The model under review builds one solid part; all positions refer to its coordinate system, in mm. Face numbers are marked on the shaded views. A direction names the side the tool comes from. Coordinates: 2 decimals unless noted, no trailing zeros. Write each loop counter-clockwise with the first axis right and the second up, starting at its lowest first coordinate (ties: lowest second). Pieces come first, ordered by that corner, then holes. Notation, with made-up numbers: (-18, -13.5) - (26, -13.5) arc R26 cw to (26, 5.5) - close; hole circle Ø7 at (-7.5, 19). An arc over 180 degrees is marked (long way). Return JSON: item names as keys, results as strings. Group by question number.
(1) For pin 1 Ø0.6 at (x, y) = (3, -1) entering from +Z; pin 2 Ø1.8 at (x, z) = (3, -4.5) entering from -Y; pin 3 Ø3 at (x, z) = (4, -3.75) entering from -Y, all flat-tipped, find the tip position at first contact; note any pin that passes through.
(2) Tool access review of the marked faces 1, 2 and 3: name each direction out of +Z, -Z, +X, -X, +Y, -Y from which nothing blocks a thin tool from reaching the whole face with its end or side.
(3) Draft analysis for pull direction X (two halves, no side actions). For the marked faces 4, 5 and 6, state which applies: released by +X, released by -X, zero draft, split by the parting line, or undercut.
(4) We need section B-B on y = 0.45. State the section outline as (x, z) points, then the cut area to 3 significant figures.
(5) We need section C-C on z = -4. State the section outline as (x, y) points.
(6) To check wall thickness, follow L1, parallel to Y at x = 2.25, z = -6; L2, parallel to Y at x = 5.5, z = -3.25; L3, parallel to X at y = 0.6, z = -3.75. State the ranges of each line that lie inside material, in increasing order. Write a range as from..to.
(7) We need section D-D on y = 2.4. State the section outline as (x, z) points.
(8) We need section A-A on x = 4. State the section outline as (y, z) points.
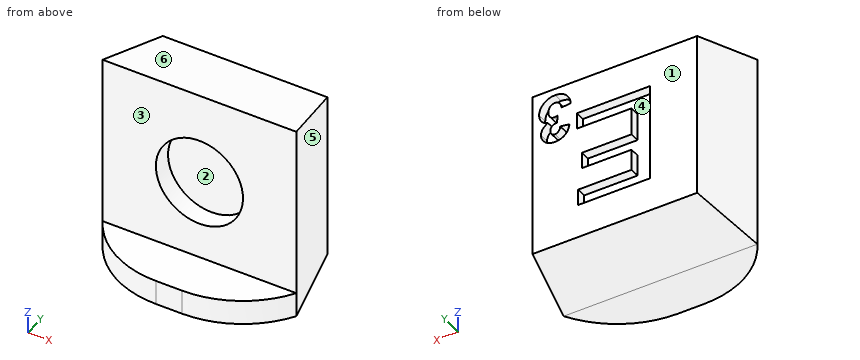
```python
from build123d import *

# Parameters (mm, degrees)
SKETCH1_W               = 8
SKETCH1_H               = 8
BOSS_EXTRUDE1_DEPTH     = 3
CUT_EXTRUDE1_DEPTH      = 12.704699911
CUT_EXTRUDE1_DEPTH_BACK = 12.704699911
CUT_EXTRUDE2_DEPTH      = 11
SKETCH4_R               = 1.8
CUT_EXTRUDE3_DEPTH      = 0.8
SKETCH5_W               = 8
SKETCH5_H               = 1
BOSS_EXTRUDE2_DEPTH     = 2
FILLET1_R               = 4
CUT_EXTRUDE4_DEPTH      = 0.4
CUT_EXTRUDE5_DEPTH      = 0.4


with BuildPart() as part:
    # Sketch1 → Boss-Extrude1 (new body)
    with BuildSketch(Plane(origin=(0, 0, 0), x_dir=(1, 0, 0), z_dir=(0, 1, 0))):
        with Locations((4, 4)):
            Rectangle(SKETCH1_W, SKETCH1_H)
    extrude(amount=BOSS_EXTRUDE1_DEPTH)

    # Sketch2 → Cut-Extrude1 (cut, two sides: drawn at the far end of the back side and taken through both)
    with BuildSketch(Plane.XY.offset(-CUT_EXTRUDE1_DEPTH_BACK)):
        Polygon((0, 0), (0.6, 3), (0, 3), align=None)
        Polygon((8, 0), (7.4, 3), (8, 3), align=None)
    extrude(amount=CUT_EXTRUDE1_DEPTH + CUT_EXTRUDE1_DEPTH_BACK, mode=Mode.SUBTRACT)

    # Sketch3 → Cut-Extrude2 (cut)
    with BuildSketch(Plane(origin=(0, 0, 0), x_dir=(0, 0, -1), z_dir=(1, 0, 0))):
        Polygon((0, 0), (0.6, 3), (0, 3), align=None)
        Polygon((8, 3), (7.4, 3), (8, 0), align=None)
    extrude(amount=CUT_EXTRUDE2_DEPTH, mode=Mode.SUBTRACT)

    # Sketch4 → Cut-Extrude3 (cut)
    with BuildSketch(Plane.XZ):
        with Locations(Location((4, -3.75, 0), (0, 0, 270))):
            Circle(SKETCH4_R)
    extrude(amount=-CUT_EXTRUDE3_DEPTH, mode=Mode.SUBTRACT)

    # Sketch5 → Boss-Extrude2 (add)
    with BuildSketch(Plane.XZ):
        with Locations((4, -7.5)):
            Rectangle(SKETCH5_W, SKETCH5_H)
    extrude(amount=BOSS_EXTRUDE2_DEPTH)

    # Fillet1
    # the kernel refuses this fillet: 4 mm, written as the material it takes off along each edge
    with BuildSketch(Plane(origin=(8, -2, -16.660254038), x_dir=(0, 1, 0), z_dir=(0, 0, 1)), Plane(origin=(0, -2, 1.660254038), x_dir=(0, 1, 0), z_dir=(0, 0, -1))) as fillet1_piece_1:
        with BuildLine():
            CenterArc((4, 3.464101615), FILLET1_R, 180, 60)
            Line((0, 3.464101615), (-0.08, 3.464101615))
            Line((-0.08, 3.464101615), (-0.08, 0))
            Line((-0.08, 0), (0, -0.08))
            ThreePointArc((0, -0.08), (1, -0.08), (1.96, -0.069282032))
            Line((1.96, -0.069282032), (2, 0))
        make_face()
    extrude(amount=18.320508076, mode=Mode.SUBTRACT)

    # Sketch6 → Cut-Extrude4 (cut)
    with BuildSketch(Plane(origin=(0, 3, 0), x_dir=(1, 0, 0), z_dir=(0, 1, 0))):
        Polygon((2.544225106, 2.010567225), (2.544225106, 6.010567225), (5.51858408, 6.010567225), (5.51858408, 5.343900558), (3.313455875, 5.343900558), (3.313455875, 4.472105686), (5.364737926, 4.472105686), (5.364737926, 3.80543902), (3.313455875, 3.80543902), (3.313455875, 2.677233891), (5.569866131, 2.677233891), (5.569866131, 2.010567225), align=None)
    extrude(amount=-CUT_EXTRUDE4_DEPTH, mode=Mode.SUBTRACT)

    # Sketch7 → Cut-Extrude5 (cut)
    with BuildSketch(Plane(origin=(0, 3, 0), x_dir=(1, 0, 0), z_dir=(0, 1, 0))):
        with BuildLine():
            Line((5.822088817, 1.468310464), (6.206704202, 1.515586105))
            add(Edge.make_bspline(
                [(6.206704202, 1.515586105), (6.210025755, 1.491936921), (6.21633053, 1.447047438), (6.235989072, 1.384914698), (6.261652315, 1.330845836), (6.295629161, 1.286544364), (6.334912115, 1.251310519), (6.37872169, 1.226169889), (6.426661607, 1.210315729), (6.460052531, 1.208713548), (6.477136894, 1.207893797)],
                knots=[0, 0, 0, 0, 1.26631894, 2.403651751, 3.447242243, 4.428907923, 5.348362865, 6.231623936, 7.095215805, 8, 8, 8, 8], degree=3))
            add(Edge.make_bspline(
                [(6.477136894, 1.207893797), (6.486366298, 1.208091994), (6.504648304, 1.20848459), (6.531523321, 1.212603697), (6.557345996, 1.219374529), (6.58186155, 1.229117251), (6.605187017, 1.241222715), (6.627629553, 1.255638676), (6.648246393, 1.273643613), (6.668375088, 1.29334292), (6.68623752, 1.315767324), (6.701972196, 1.340096861), (6.715784117, 1.366090219), (6.726489771, 1.394417604), (6.734869896, 1.424465406), (6.740860884, 1.456364057), (6.744506994, 1.489993317), (6.74494315, 1.513039367), (6.74516574, 1.524800849)],
                knots=[0, 0, 0, 0, 0.951760839, 1.885289532, 2.797832748, 3.70117291, 4.60103766, 5.506897018, 6.445598779, 7.420035506, 8.410036365, 9.396193293, 10.407074535, 11.440988179, 12.514285005, 13.622404236, 14.786601276, 16, 16, 16, 16], degree=3))
            add(Edge.make_bspline(
                [(6.74516574, 1.524800849), (6.744331981, 1.546629456), (6.742741494, 1.588269906), (6.730451294, 1.647346431), (6.709137892, 1.699277092), (6.679276772, 1.743130281), (6.643793264, 1.778406879), (6.604044422, 1.8049236), (6.559654571, 1.820157256), (6.528795478, 1.822230353), (6.513194586, 1.823278413)],
                knots=[0, 0, 0, 0, 1.241512862, 2.368321189, 3.414110003, 4.41529485, 5.36642979, 6.245396713, 7.112955941, 8, 8, 8, 8], degree=3))
            add(Edge.make_bspline(
                [(6.513194586, 1.823278413), (6.502087722, 1.822994208), (6.47854234, 1.822391724), (6.441918774, 1.81613185), (6.401980616, 1.80749294), (6.374785766, 1.799182881), (6.360550356, 1.7948329)],
                knots=[0, 0, 0, 0, 0.854525515, 1.811503923, 2.854410343, 4, 4, 4, 4], degree=3))
            Line((6.360550356, 1.7948329), (6.396608048, 2.105329695))
            add(Edge.make_bspline(
                [(6.396608048, 2.105329695), (6.407296254, 2.105146348), (6.428036665, 2.104790564), (6.458323888, 2.107301653), (6.486673662, 2.111886341), (6.513019839, 2.119324972), (6.53738695, 2.128349551), (6.559988104, 2.139688262), (6.580270378, 2.153798702), (6.604965361, 2.175098338), (6.630230561, 2.207014566), (6.6530719, 2.250778884), (6.665798637, 2.300679459), (6.667408863, 2.335629458), (6.668242663, 2.353727131)],
                knots=[0, 0, 0, 0, 0.916749589, 1.778948191, 2.604102396, 3.376994206, 4.124053722, 4.831292757, 5.54010828, 6.238660037, 7.62386988, 9.002523041, 10.447858069, 12, 12, 12, 12], degree=3))
            add(Edge.make_bspline(
                [(6.668242663, 2.353727131), (6.667680515, 2.36913782), (6.666602635, 2.398686702), (6.656933325, 2.440733393), (6.640429824, 2.477855418), (6.617345194, 2.50940841), (6.589028098, 2.535030406), (6.555929861, 2.553963194), (6.518019093, 2.565003531), (6.491366313, 2.566231188), (6.477537535, 2.566868156)],
                knots=[0, 0, 0, 0, 1.146968804, 2.199229744, 3.192297141, 4.153502289, 5.090509175, 6.0173182, 6.971286811, 8, 8, 8, 8], degree=3))
            add(Edge.make_bspline(
                [(6.477537535, 2.566868156), (6.463673911, 2.566182836), (6.436422829, 2.564835732), (6.397428508, 2.551510744), (6.361454157, 2.530893795), (6.329709376, 2.501368407), (6.302195486, 2.464646404), (6.280874208, 2.419861118), (6.265858745, 2.367714197), (6.260698213, 2.33018187), (6.257986253, 2.3104579)],
                knots=[0, 0, 0, 0, 0.889956214, 1.749345552, 2.62404616, 3.543272128, 4.520224035, 5.562553653, 6.719074424, 8, 8, 8, 8], degree=3))
            Line((6.257986253, 2.3104579), (5.873370869, 2.368150208))
            add(Edge.make_bspline(
                [(5.873370869, 2.368150208), (5.879712758, 2.397514751), (5.891852554, 2.453725064), (5.916656, 2.532479948), (5.945759151, 2.602002338), (5.979761878, 2.663071325), (6.020038823, 2.716762155), (6.067859884, 2.763365742), (6.122509575, 2.804234412), (6.183883545, 2.838478774), (6.250614825, 2.865925856), (6.321633047, 2.886240153), (6.396757082, 2.897882068), (6.448117417, 2.899417689), (6.474332407, 2.90020149)],
                knots=[0, 0, 0, 0, 1.220808349, 2.336900656, 3.3513467, 4.279992853, 5.171472476, 6.069835959, 6.985198729, 7.938095762, 8.919113729, 9.91246339, 10.934493858, 12, 12, 12, 12], degree=3))
            add(Edge.make_bspline(
                [(6.474332407, 2.90020149), (6.496795991, 2.899690329), (6.540685792, 2.898691614), (6.604687523, 2.890097866), (6.665244055, 2.876137228), (6.722439804, 2.856388937), (6.776539911, 2.831244798), (6.826641223, 2.799609265), (6.873794781, 2.763093379), (6.901724377, 2.73467508), (6.915838817, 2.720313669)],
                knots=[0, 0, 0, 0, 1.096978699, 2.143298912, 3.148181587, 4.128190255, 5.094201205, 6.055441919, 7.017302331, 8, 8, 8, 8], degree=3))
            add(Edge.make_bspline(
                [(6.915838817, 2.720313669), (6.926741328, 2.708075606), (6.948274918, 2.683904162), (6.976233385, 2.645150995), (6.999633117, 2.604882958), (7.019482141, 2.563940258), (7.034243104, 2.52137348), (7.04524752, 2.477850813), (7.051783755, 2.43298662), (7.05249893, 2.402626167), (7.052858048, 2.387380977)],
                knots=[0, 0, 0, 0, 1.065582675, 2.104636323, 3.101288825, 4.092056841, 5.059084899, 6.026073946, 7.008813224, 8, 8, 8, 8], degree=3))
            add(Edge.make_bspline(
                [(7.052858048, 2.387380977), (7.052074688, 2.365937591), (7.050530541, 2.323668734), (7.036361111, 2.262180096), (7.013586987, 2.204054017), (6.982096895, 2.149068456), (6.941041129, 2.097733658), (6.890499978, 2.050511525), (6.831958555, 2.005600039), (6.787958464, 1.980231405), (6.765197792, 1.967108541)],
                knots=[0, 0, 0, 0, 0.957571776, 1.887550067, 2.804499428, 3.740591036, 4.709432777, 5.731457079, 6.826512349, 8, 8, 8, 8], degree=3))
            add(Edge.make_bspline(
                [(6.765197792, 1.967108541), (6.778741549, 1.963844189), (6.805468134, 1.957402478), (6.844077906, 1.94426987), (6.880236126, 1.927424278), (6.914828375, 1.908914943), (6.946996208, 1.886966635), (6.977363151, 1.862646466), (7.00476785, 1.834549826), (7.03102769, 1.804865641), (7.053982146, 1.772288453), (7.074722978, 1.738388398), (7.091382436, 1.702338355), (7.105631297, 1.665065232), (7.116248441, 1.625966572), (7.124562393, 1.585334894), (7.128729622, 1.542917296), (7.129427921, 1.514124194), (7.129781125, 1.499560464)],
                knots=[0, 0, 0, 0, 1.037381978, 2.047118658, 3.030848314, 4.005687143, 4.965748246, 5.927353932, 6.897971669, 7.885165084, 8.876109723, 9.862099733, 10.840989857, 11.829385213, 12.830906716, 13.855042526, 14.915067134, 16, 16, 16, 16], degree=3))
            add(Edge.make_bspline(
                [(7.129781125, 1.499560464), (7.129332308, 1.478289376), (7.12844718, 1.43633993), (7.11872513, 1.374773186), (7.10395436, 1.3156035), (7.083598929, 1.25859183), (7.056376257, 1.204435717), (7.023823759, 1.152375398), (6.985054773, 1.102929453), (6.940845684, 1.056472589), (6.892539484, 1.013951446), (6.84063463, 0.97660242), (6.785900139, 0.944991177), (6.728022396, 0.9191431), (6.667504686, 0.899031537), (6.603826037, 0.885208987), (6.537502989, 0.875987213), (6.49212598, 0.875040406), (6.469124074, 0.874560464)],
                knots=[0, 0, 0, 0, 1.006520189, 1.984993146, 2.943645202, 3.891894145, 4.845023195, 5.808336607, 6.795092628, 7.815033679, 8.841288157, 9.838185905, 10.83832808, 11.829129029, 12.835072876, 13.85234392, 14.911338897, 16, 16, 16, 16], degree=3))
            add(Edge.make_bspline(
                [(6.469124074, 0.874560464), (6.447326457, 0.874925903), (6.404510806, 0.875643711), (6.341832261, 0.884147308), (6.281800208, 0.896657101), (6.224765045, 0.914957582), (6.170229951, 0.937498647), (6.119224255, 0.966556317), (6.070434994, 0.999582769), (6.02545616, 1.03827062), (5.983635573, 1.080436419), (5.946901196, 1.126807021), (5.914165969, 1.175902437), (5.886010541, 1.228157933), (5.862670856, 1.283709297), (5.844497682, 1.342413141), (5.830004226, 1.404089696), (5.824763645, 1.446608551), (5.822088817, 1.468310464)],
                knots=[0, 0, 0, 0, 1.077528213, 2.11651914, 3.123276654, 4.10732375, 5.075386463, 6.036572488, 7.005896639, 7.98540975, 8.966414275, 9.939311093, 10.906719916, 11.882103104, 12.870994428, 13.882228509, 14.919075059, 16, 16, 16, 16], degree=3))
        make_face()
    extrude(amount=-CUT_EXTRUDE5_DEPTH, mode=Mode.SUBTRACT)


solid = part.part
```
Ans:
{
 "1": {"pin 1": "z = -7", "pin 2": "y = 0", "pin 3": "y = 0.8"},
 "2": {"face 1": "+Z, -Z, +X, -X, +Y", "face 2": "-Y", "face 3": "+Z, +X, -X, -Y"},
 "3": {"face 4": "undercut", "face 5": "released by +X", "face 6": "zero draft"},
 "4": {"outline": "(0.09, -7.91) - (7.91, -7.91) - (7.91, -0.09) - (0.09, -0.09) - close; hole circle Ø3.6 at (4, -3.75)", "area": "51.0 mm²"},
 "5": {"outline": "(0, 0) - (2.22, 0) - (2.22, 0.8) - (5.78, 0.8) - (5.78, 0) - (8, 0) - (7.4, 3) - (5.36, 3) - (5.36, 2.6) - (2.54, 2.6) - (2.54, 3) - (0.6, 3) - close"},
 "6": {"L1": "0..3", "L2": "0.8..3", "L3": "0.12..2.2, 5.8..7.88"},
 "7": {"outline": "(0.48, -7.52) - (7.52, -7.52) - (7.52, -0.48) - (0.48, -0.48) - close"},
 "8": {"outline": "(-2, -8) - (0, -8) - (3, -7.4) - (3, -6.01) - (2.6, -6.01) - (2.6, -5.34) - (3, -5.34) - (3, -4.47) - (2.6, -4.47) - (2.6, -3.81) - (3, -3.81) - (3, -2.68) - (2.6, -2.68) - (2.6, -2.01) - (3, -2.01) - (3, -0.6) - (0, 0) - (0, -1.95) - (0.8, -1.95) - (0.8, -5.55) - (0, -5.55) - (0, -7) - (-2, -7) - close"}
}
